Autodesk Inventor part; units mm, degrees
ref_plane "YZ Plane" through (0, 0, 0) normal (1, 0, 0) x (0, 1, 0)
ref_plane "XZ Plane" through (0, 0, 0) normal (0, 1, 0) x (-1, 0, 0)
ref_plane "XY Plane" through (0, 0, 0) normal (0, 0, 1) x (1, 0, 0)
sketch "Sketch1" plane through (0, 0, 0) normal (0, 0, 1) x (1, 0, 0)
  line L0 (0, 0) -> (-127, 0)
  line L1 (-127, 0) -> (-127, 101.6)
  line L2 (-127, 101.6) -> (0, 101.6)
  line L3 (0, 101.6) -> (0, 0)
  dimension "d0" = 127
  dimension "d1" = 101.6
extrude "Extrusion1" add sketch "Sketch1" along normal blind 1.5875
sketch "Sketch3" plane through (0, 0, 1.5875) normal (0, 0, 1) x (1, 0, 0)
  line L0 (0, 101.6) -> (-127, 101.6)
  line L1 (-6.35, 101.6) -> (-6.35, 95.25)
  line L2 (-6.35, 95.25) -> (0, 95.25)
  line L3 (0, 0) -> (0, 101.6)
  line L4 (-6.35, 95.25) -> (-44.45, 95.25)
  line L5 (-44.45, 95.25) -> (-82.55, 95.25)
  line L6 (-82.55, 95.25) -> (-120.65, 95.25)
  line L7 (-120.65, 95.25) -> (-127, 95.25)
  line L8 (-120.65, 95.25) -> (-120.65, 19.05)
  line L9 (-120.65, 19.05) -> (-120.65, 6.35)
  circle A0 centre (-120.65, 19.05) radius 2.54
  circle A1 centre (-120.65, 6.35) radius 2.54
  line L10 (-6.35, 95.25) -> (-6.35, 19.05)
  circle A2 centre (-6.35, 19.05) radius 2.54
  line L11 (-6.35, 19.05) -> (-6.35, 6.35)
  circle A3 centre (-6.35, 6.35) radius 2.54
  line L12 (-6.35, 6.35) -> (-57.15, 6.35)
  circle A4 centre (-57.15, 6.35) radius 2.54
  line L13 (-57.15, 6.35) -> (-69.85, 6.35)
  circle A5 centre (-69.85, 6.35) radius 2.54
  line L14 (-69.85, 6.35) -> (-120.65, 6.35)
  line L15 (-69.85, 6.35) -> (-69.85, 19.05)
  line L16 (-57.15, 6.35) -> (-57.15, 19.05)
  circle A6 centre (-69.85, 19.05) radius 2.54
  circle A7 centre (-57.15, 19.05) radius 2.54
  line L17 (-120.65, 95.25) -> (-107.9525, 95.25)
  line L18 (-101.6, 95.25) -> (-95.25, 95.25)
  line L19 (-95.25, 95.25) -> (-95.25, 54.61)
  circle A8 centre (-95.25, 54.61) radius 5.08
  line L20 (-25.4, 95.25) -> (-31.75, 95.25)
  line L21 (-44.45, 95.25) -> (-31.75, 95.25)
  line L22 (-31.75, 95.25) -> (-31.75, 54.61)
  circle A9 centre (-31.75, 54.61) radius 5.08
  line L23 (-120.65, 95.25) -> (-120.65, 97.79)
  line L24 (-6.35, 95.25) -> (-6.35, 97.79)
  line L25 (-82.55, 95.25) -> (-82.55, 97.79)
  line L26 (-44.45, 95.25) -> (-44.45, 97.79)
  line L27 (-120.65, 97.79) -> (-120.65, 96.52)
  line L28 (-82.55, 97.79) -> (-82.55, 96.52)
  line L29 (-44.45, 97.79) -> (-44.45, 96.52)
  line L30 (-6.35, 97.79) -> (-6.35, 96.52)
  line L31 (-120.65, 96.52) -> (-120.65, 94.9198)
  circle A10 centre (-120.65, 94.9198) radius 2.54
  line L32 (-82.55, 96.52) -> (-82.55, 94.9198)
  circle A11 centre (-82.55, 94.9198) radius 2.54
  line L33 (-44.45, 96.52) -> (-44.45, 94.9198)
  line L34 (-6.35, 96.52) -> (-6.35, 94.9198)
  circle A12 centre (-6.35, 94.9198) radius 2.54
  circle A13 centre (-44.45, 94.9198) radius 2.54
  dimension "d4" = 6.35
  dimension "d5" = 6.35
  dimension "d7" = 38.1
  dimension "d8" = 38.1
  dimension "d9" = 38.1
  dimension "d10" = 6.35
  dimension "d20" = 76.2
  dimension "d21" = 12.7
  dimension "d22" = 5.08
  dimension "d23" = 5.08
  dimension "d26" = 76.2
  dimension "d27" = 5.08
  dimension "d28" = 12.7
  dimension "d29" = 5.08
  dimension "d33" = 50.8
  dimension "d34" = 5.08
  dimension "d35" = 12.7
  dimension "d36" = 5.08
  dimension "d37" = 12.7
  dimension "d38" = 5.08
  dimension "d39" = 5.08
  dimension "d41" = 10.16
  dimension "d42" = 10.16
  dimension "d43" = 40.64
  dimension "d44" = 40.64
  dimension "d53" = 1.6002
  dimension "d54" = 5.08
  dimension "d55" = 1.6002
  dimension "d56" = 5.08
  dimension "d57" = 1.6002
  dimension "d58" = 1.6002
  dimension "d59" = 5.08
  dimension "d60" = 5.08
extrude "Extrusion2" cut sketch "Sketch3" against normal blind 25.4 contours A12 L10 L2 | L2 L1 A12 | L1 L4 A12 | L10 A12 L4 | A9 | A8 | A6 | A7 | A2 L11 L10 | L10 L11 A2 | A13 L5 L4 | L4 L26 A13 | A3 L12 L11 | L11 L12 A3 | L5 A13 L26 | A4 L13 L12 | L12 L16 A4 | A11 L6 L5 | L5 L25 A11 | L13 A4 L16 | L6 A11 L25 | A5 L14 L13 | L13 L15 A5 | L14 A5 L15 | L14 L9 A1 | A1 L9 L14 | A0 L8 L9 | L9 L8 A0 | A10 L8 L6 | L6 L23 A10 | L8 A10 L7 | L7 A10 L23
fillet "Fillet1" radius 3.175 4 edges at (-127, 101.6, 0.7937) (0, 101.6, 0.7937) (0, 0, 0.7937) (-127, 0, 0.7937)
properties part number "Polycarbonate Kicker plate"
Source: CAD feature listing. Evaluate the final solid. Frame: model axes, mm. Coordinates: 2 decimals unless noted, no trailing zeros. Loops run counter-clockwise (first coordinate to the right, second up) from the corner with the lowest first, then second, coordinate; pieces in that order, holes last. Notation, with made-up numbers: M 74.25,12.5 L 119.25,12.5 A25 cw 119.25,27.5 Z; hole C 23.5,-17 d7. An arc over 180 degrees is marked long. Use CSV: the item, a comma, the result in double quotes.
(1) Cut plane D-D on x = -82.55. Return loops of the section in (y, z), and give its area (3 significant figures).
Answers follow:
outline,"M 0,0 L 92.38,0 L 92.38,1.59 L 0,1.59 Z; M 97.46,0 L 101.6,0 L 101.6,1.59 L 97.46,1.59 Z"
area,"153 mm²"
(2) Cut plane A-A on y = 6.35. Return loops of the section in (x, z).
Answers follow:
outline,"M -127,0 L -123.19,0 L -123.19,1.59 L -127,1.59 Z; M -118.11,0 L -72.39,0 L -72.39,1.59 L -118.11,1.59 Z; M -67.31,0 L -59.69,0 L -59.69,1.59 L -67.31,1.59 Z; M -54.61,0 L -8.89,0 L -8.89,1.59 L -54.61,1.59 Z; M -3.81,0 L 0,0 L 0,1.59 L -3.81,1.59 Z"
(3) Draft query along Y for faces 1 (the face through (-0.95, 0.91, 0.8)), 2 (the face through (-72.388, 6.462, 0.805)), 3 (the face through (-126.05, 100.69, 0.8)). Return one class per face: pulls with the +Y half, pulls with the -Y half, needs draft (parallel to the pull), parting line crosses it, or undercut.
Answers follow:
face 1,"pulls with the -Y half"
face 2,"undercut"
face 3,"pulls with the +Y half"
(4) Line query: line 1 (Y direction, x = -57.15, z = 0.85); line 2 (X direction, y = 19.05, z = 0.7); line 3 (X direction, y = 54.61, z = 0.3). Output: solid intervals per line, ascending. Write a range as [from, to].
Answers follow:
line 1,"[0, 3.81], [8.89, 16.51], [21.59, 101.6]"
line 2,"[-127, -123.19], [-118.11, -72.39], [-67.31, -59.69], [-54.61, -8.89], [-3.81, 0]"
line 3,"[-127, -100.33], [-90.17, -36.83], [-26.67, 0]"
(5) Cut plane C-C on y = 54.61. Return loops of the section in (x, z), and give its area (3 significant figures).
Answers follow:
outline,"M -127,0 L -100.33,0 L -100.33,1.59 L -127,1.59 Z; M -90.17,0 L -36.83,0 L -36.83,1.59 L -90.17,1.59 Z; M -26.67,0 L 0,0 L 0,1.59 L -26.67,1.59 Z"
area,"169 mm²"
(6) Cut plane B-B on x = -31.75. Return loops of the section in (y, z), and give its area (3 significant figures).
Answers follow:
outline,"M 0,0 L 49.53,0 L 49.53,1.59 L 0,1.59 Z; M 59.69,0 L 101.6,0 L 101.6,1.59 L 59.69,1.59 Z"
area,"145 mm²"
